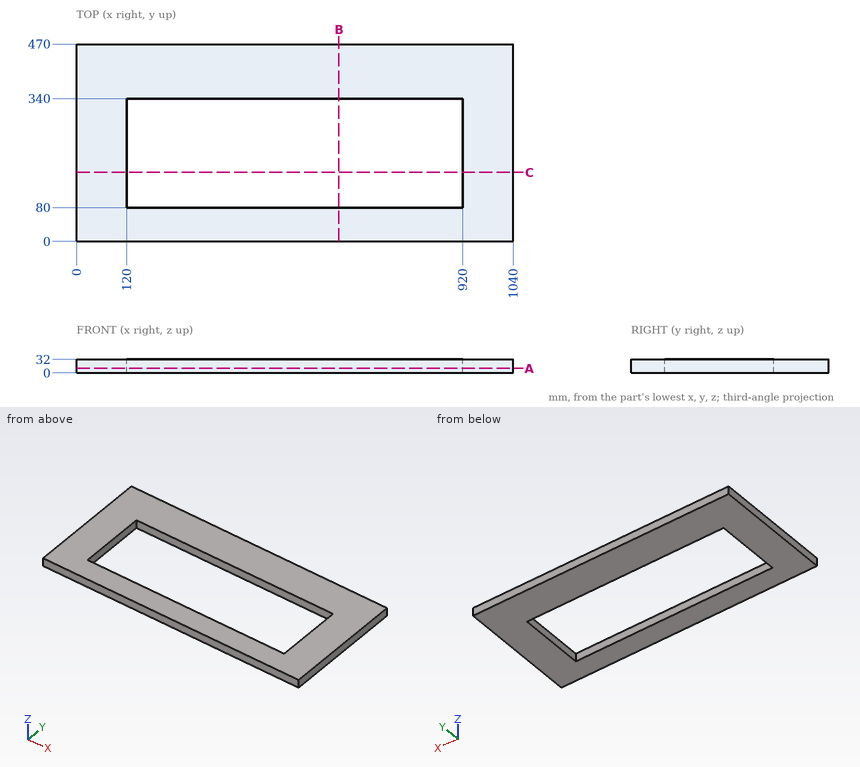
Verification items for this drawing (mm, ordinates from the low corner). Give positions to 0.01 mm unless a question says otherwise; leave off trailing zeros. Loops run counter-clockwise (first coordinate to the right, second up) from the corner with the lowest first, then second, coordinate; pieces in that order, holes last.
1. Cross-section at C-C on y = 164.5. Record the cut outline in (x, z), and give its area (3 significant figures).
Derived:
outline: (0, 0) - (120, 0) - (120, 32) - (0, 32) - close; (920, 0) - (1040, 0) - (1040, 32) - (920, 32) - close
area: 7,680 mm2
2. Material ranges on probe 1 along Y at (x, z) = (725, 19.5); probe 2 along X at (y, z) = (332.5, 11), recorded low to high.
Derived:
probe 1: y = 0 to 80, 340 to 470
probe 2: x = 0 to 120, 920 to 1040
3. Cross-section at A-A on z = 10.5. Record the cut outline in (x, y).
Derived:
outline: (0, 0) - (1040, 0) - (1040, 470) - (0, 470) - close; hole (120, 80) - (920, 80) - (920, 340) - (120, 340) - close
4. Cross-section at B-B on x = 625. Record the cut outline in (y, z), and give its area (3 significant figures).
Derived:
outline: (0, 0) - (80, 0) - (80, 32) - (0, 32) - close; (340, 0) - (470, 0) - (470, 32) - (340, 32) - close
area: 6,720 mm2
